from build123d import *

# Parameters (mm, degrees)
F1_DEPTH = 25


with BuildPart() as f1:
    # F0 (on Front) → F1 (new body)
    with BuildSketch(Plane.XZ):
        Polygon((367.473159, 37.881499), (63.624065, 37.881499), (22.529194, 26.785146), (-74.708393, 26.785146), (-109.664981, 37.881499), (-135.774802, 12.936393), (-281.499266, 5.046134), (-318.647265, -6.34683), (-282.593813, -87.8235), (-227.826428, -87.8235), (-215.265799, -64.971001), (-211.985035, -42.118501), (-210.623877, -32.637216), (-136.59613, -32.637216), (-128.112047, -32.177844), (-133.220164, -42.118501), (-109.659574, -42.118501), (-93.017144, -42.118501), (-87.93899, -42.118501), (156.094849, 0), (405.345833, 0), align=None)
        Polygon((-122.766047, -66.823296), (-109.659574, -42.118501), (-133.220164, -42.118501), (-148.813925, -72.464758), (-151.375101, -77.448938), (-158.60486, -91.51842), (-140.738134, -100.699436), (-125.198854, -71.408968), align=None)
        with BuildLine():
            ThreePointArc((-121.31966, -72.286692), (-97.447394, -65.149299), (-87.93899, -42.118501))
            Line((-87.93899, -42.118501), (-93.017144, -42.118501))
            ThreePointArc((-93.017144, -42.118501), (-92.994342, -44.768054), (-93.264839, -47.403862))
            ThreePointArc((-93.264839, -47.403862), (-102.08842, -62.436086), (-118.771899, -67.484341))
            ThreePointArc((-118.771899, -67.484341), (-120.782989, -67.238505), (-122.766047, -66.823296))
            Line((-122.766047, -66.823296), (-125.198854, -71.408968))
            ThreePointArc((-125.198854, -71.408968), (-123.274332, -71.914456), (-121.31966, -72.286692))
        make_face()
        with BuildLine():
            ThreePointArc((-93.264839, -47.403862), (-92.994342, -44.768054), (-93.017144, -42.118501))
            Line((-93.017144, -42.118501), (-109.659574, -42.118501))
            Line((-109.659574, -42.118501), (-122.766047, -66.823296))
            ThreePointArc((-122.766047, -66.823296), (-120.782989, -67.238505), (-118.771899, -67.484341))
            Line((-118.771899, -67.484341), (-108.118735, -47.403862))
            Line((-108.118735, -47.403862), (-93.264839, -47.403862))
        make_face()
        Polygon((-135.613307, -38.852425), (-133.220164, -42.118501), (-128.112047, -32.177844), (-136.59613, -32.637216), (-210.623877, -32.637216), (-211.985035, -42.118501), (-215.265799, -64.971001), (-158.870872, -75.985004), (-151.375101, -77.448938), (-148.813925, -72.464758), (-152.885377, -72.464758), (-161.944241, -70.69555), (-206.79819, -61.935515), (-203.630078, -38.852425), (-145.581298, -38.852425), align=None)
        with BuildLine():
            Line((-137.324025, -102.453814), (-121.31966, -72.286692))
            ThreePointArc((-121.31966, -72.286692), (-123.274332, -71.914456), (-125.198854, -71.408968))
            Line((-125.198854, -71.408968), (-140.738134, -100.699436))
            Line((-140.738134, -100.699436), (-137.324025, -102.453814))
        make_face()
    extrude(amount=F1_DEPTH)


solid = f1.part
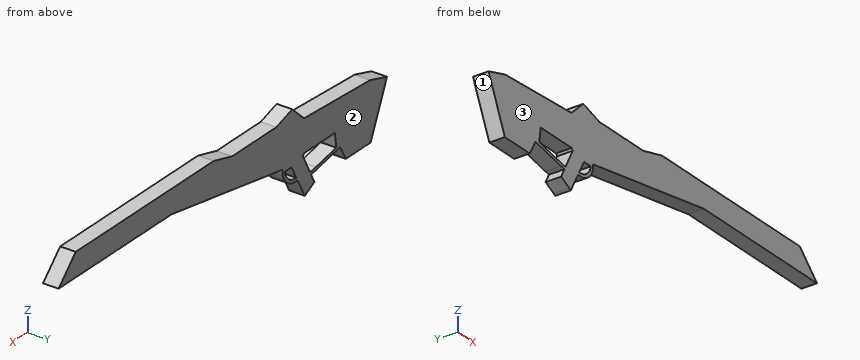
Here's how the part is built. I have some questions about the finished solid (model axes, mm). Face numbers are marked on the shaded views. Round coordinates to 2 decimals unless told otherwise and drop trailing zeros. Order: outer loops, then holes, each group sorted by start corner. A loop starts at its lowest first (then second) coordinate and runs counter-clockwise, first axis right, second up. Notation, with made-up numbers: (48.25, 33) -> (80.25, 33) arc R14 cw to (80.25, 51) -> close; hole circle Ø6 at (50.5, -30). An arc over 180 degrees is marked (long way). Return JSON: item names as keys, results as strings.
Q1. If we section it at A-A on y = -13.25: List the corners of the cut face in (x, z) for me (1 decimal).
Filled sheet:
{"outline": "(-318.6, -6.3) -> (-282.6, -87.8) -> (-227.8, -87.8) -> (-215.3, -65) -> (-151.4, -77.4) -> (-158.6, -91.5) -> (-137.3, -102.5) -> (-121.3, -72.3) arc R29 ccw to (-87.9, -42.1) -> (156.1, 0) -> (405.3, 0) -> (367.5, 37.9) -> (63.6, 37.9) -> (22.5, 26.8) -> (-74.7, 26.8) -> (-109.7, 37.9) -> (-135.8, 12.9) -> (-281.5, 5) -> close; hole (-206.8, -61.9) -> (-152.9, -72.5) -> (-148.8, -72.5) -> (-133.2, -42.1) -> (-135.6, -38.9) -> (-203.6, -38.9) -> close; hole (-118.8, -67.5) arc R23.9 ccw to (-93.3, -47.4) -> (-108.1, -47.4) -> close"}
Q2. For pin 1 Ø12 at (x, y) = (7, -10.5) entering from -Z; pin 2 Ø2 at (x, y) = (-151, -7) entering from +Z; pin 3 Ø10 at (x, y) = (-124, -14.5) entering from +Z, each with a flat end and sliding along its axis, tell me the tip position at first contact or that it passes through.
Filled sheet:
{"pin 1": "stops at z = -26.77", "pin 2": "stops at z = 12.17", "pin 3": "stops at z = 28.96"}
Q3. If we section it at C-C on z = -15: List the corners of the cut face in (x, y) for me, plus the area to 3 significant figures.
Filled sheet:
{"outline": "(-314.82, -25) -> (69.19, -25) -> (69.19, 0) -> (-314.82, 0) -> close", "area": "9,600 mm^2"}
Q4. If we section it at B-B on x = 223.5: List the corners of the cut face in (y, z) for me.
Filled sheet:
{"outline": "(-25, 0) -> (0, 0) -> (0, 37.88) -> (-25, 37.88) -> close"}
Q5. I need wall thicknesses on line 1 along X through (y, z) = (-8.25, -61.5); line 2 along X through (y, z) = (-15.5, -51.5); line 3 along Z through (x, y) = (236, -3.25). Which ranges of each line are inside material? Lowest first, please. Write a range as from..to.
Filled sheet:
{"line 1": "x = -294.24..-206.74, -143.18..-115.6, -100.97..-94.05", "line 2": "x = -298.67..-205.37, -138.04..-110.29, -94.29..-88.98", "line 3": "z = 0..37.88"}
Q6. If we mould it in two halves opening along Y, with no side actions, what happens to the marked faces 1, 2 and 3? For each: released by +Y, released by -Y, zero draft, split by the parting line, or undercut.
Filled sheet:
{"face 1": "zero draft", "face 2": "released by +Y", "face 3": "released by -Y"}
